Model file for the job. Use its own axes, mm. A direction names the side the tool comes from. Round coordinates to 2 decimals unless told otherwise and drop trailing zeros. Order: outer loops, then holes, each group sorted by start corner. A loop starts at its lowest first (then second) coordinate and runs counter-clockwise, first axis right, second up. Notation, with made-up numbers: (35, 64.25) - (75, 64.25) arc R22 cw to (75, 83.25) - close; hole circle Ø1 at (65.25, 16). An arc over 180 degrees is marked (long way). Write item = value, one per line.
```python
from build123d import *

# Parameters (mm, degrees)
SKETCH1_W           = 6
SKETCH1_H           = 3
BOSS_EXTRUDE1_DEPTH = 15
SKETCH2_R           = 0.75
CUT_EXTRUDE1_DEPTH  = 20
CHAMFER1_SIZE       = 0.6
SKETCH3_R           = 1
CUT_EXTRUDE2_DEPTH  = 20
LPATTERN1_COUNT     = 4
LPATTERN1_PITCH     = 3.5
SKETCH4_W           = 3.6
SKETCH4_H           = 1.5
CUT_EXTRUDE3_DEPTH  = 20
CHAMFER2_SIZE       = 0.5


with BuildPart() as part:
    # Sketch1 → Boss-Extrude1 (new body)
    with BuildSketch(Plane.XY):
        Rectangle(SKETCH1_W, SKETCH1_H)
    extrude(amount=BOSS_EXTRUDE1_DEPTH)

    # Sketch2 → Cut-Extrude1 (cut)
    with BuildSketch(Plane.XY.offset(15)):
        with Locations((3, 0)):
            Circle(SKETCH2_R)
        with Locations((-3, 0)):
            Circle(SKETCH2_R)
    extrude(amount=-CUT_EXTRUDE1_DEPTH, mode=Mode.SUBTRACT)

    # Chamfer1
    chamfer1_edges = [part.edges().sort_by_distance(p)[0] for p in [
        (3, -1.5, 7.5),
        (-3, -1.5, 7.5),
    ]]
    chamfer(chamfer1_edges, length=CHAMFER1_SIZE)

    # Sketch3 → Cut-Extrude2 (cut)
    with BuildSketch(Plane(origin=(0, 1.5, 0), x_dir=(1, 0, 0), z_dir=(0, 1, 0))):
        with Locations((0, -2.5)):
            Circle(SKETCH3_R)
    cut_extrude2 = extrude(amount=-CUT_EXTRUDE2_DEPTH, mode=Mode.SUBTRACT)

    # LPattern1: Cut-Extrude2 ×4
    with Locations(*[(0, 0, i * LPATTERN1_PITCH) for i in range(1, LPATTERN1_COUNT)]):
        add(cut_extrude2, mode=Mode.SUBTRACT)

    # Sketch4 → Cut-Extrude3 (cut)
    with BuildSketch(Plane(origin=(0, 0, 0), x_dir=(-1, 0, 0), z_dir=(0, 0, -1))):
        with Locations((0, -0.75)):
            Rectangle(SKETCH4_W, SKETCH4_H)
    extrude(amount=-CUT_EXTRUDE3_DEPTH, mode=Mode.SUBTRACT)

    # Chamfer2
    chamfer2_edges = [part.edges().sort_by_distance(p)[0] for p in [
        (1.8, 0, 7.5),
        (-1.8, 0, 7.5),
    ]]
    chamfer(chamfer2_edges, length=CHAMFER2_SIZE)


solid = part.part
```
1) Mould opens along Z. For faces 1 (the face through (0, 1, 14)), 2 (the face through (-0.13, 0.76, 8.51)), 3 (the face through (0, 0.4, 0)), 4 (the face through (-2.25, -0.02, 7.6)) say: +Z half, -Z half, draft (parallel to the pull), parting line (faces both ways), or undercut.
Conclusion:
face_1 = undercut
face_2 = undercut
face_3 = -Z half
face_4 = draft
2) Cut at D-D (y = -0.25). Write the cut outline in (x, z), and give its area (3 significant figures).
Conclusion:
outline = (-2.29, 0) - (-1.55, 0) - (-1.55, 15) - (-2.29, 15) - close; (1.55, 0) - (2.29, 0) - (2.29, 15) - (1.55, 15) - close
area = 22.3 mm^2
3) Cut at C-C (x = -0.75). Write the cut outline in (y, z).
Conclusion:
outline = (0, 0) - (1.5, 0) - (1.5, 1.84) - (0, 1.84) - close; (0, 3.16) - (1.5, 3.16) - (1.5, 5.34) - (0, 5.34) - close; (0, 6.66) - (1.5, 6.66) - (1.5, 8.84) - (0, 8.84) - close; (0, 10.16) - (1.5, 10.16) - (1.5, 12.34) - (0, 12.34) - close; (0, 13.66) - (1.5, 13.66) - (1.5, 15) - (0, 15) - close
4) Wall check: line 1 along Z through (x, y) = (0, 0.4); line 2 along X through (y, z) = (1.1, 2.5); line 3 along X through (y, z) = (-1.1, 10). Give the ranges that are in metal, low to high.
Conclusion:
line_1 = 0 to 1.5, 3.5 to 5, 7 to 8.5, 10.5 to 12, 14 to 15
line_2 = -3 to -1, 1 to 3
line_3 = -2.8 to -1.8, 1.8 to 2.8
5) Flat gauge pins, fed straight in: pin 1 Ø3 at (x, z) = (0, 9.5) entering from -Y; pin 2 Ø2.5 at (x, z) = (0, 6) entering from -Y. Where does each tip first touch, or does it go through?
Conclusion:
pin_1 = -0.2
pin_2 = 0
6) Cut at A-A (z = 2.5). Write the cut outline in (x, y).
Conclusion:
outline = (-3, -0.9) - (-2.4, -1.5) - (-1.8, -1.5) - (-1.8, -0.5) - (-1.3, 0) - (-1, 0) - (-1, 1.5) - (-3, 1.5) - (-3, 0.75) arc R0.75 cw to (-3, -0.75) - close; (1, 0) - (1.3, 0) - (1.8, -0.5) - (1.8, -1.5) - (2.4, -1.5) - (3, -0.9) - (3, -0.75) arc R0.75 cw to (3, 0.75) - (3, 1.5) - (1, 1.5) - close
7) 3-axis set-ups, long thin cutter, end or side, ignore diameter. For faces 5 (the face through (0, 0, 7.4)), 6 (the face through (0, 0.4, 15)): which of +Z, -Z, +X, -X, +Y, -Y reach the whole face in a straight line?
Conclusion:
face_5 = +Z, -Z, -Y
face_6 = +Z, +X, -X, +Y, -Y
8) Cut at B-B (y = 1.1). Write the cut outline in (x, z), and give its area (3 significant figures).
Conclusion:
outline = (-3, 0) - (3, 0) - (3, 15) - (-3, 15) - close; hole circle Ø2 at (0, 2.5); hole circle Ø2 at (0, 6); hole circle Ø2 at (0, 9.5); hole circle Ø2 at (0, 13)
area = 77.4 mm^2
